from build123d import *

# Parameters (mm, degrees)
BOSS_EXTRUDE1_DEPTH = 40
BOSS_EXTRUDE2_REACH = 105.634
SKETCH2_R           = 18
SKETCH3_R           = 15
SKETCH3_R_2         = 10
BOSS_EXTRUDE3_DEPTH = 18
BOSS_EXTRUDE5_DEPTH = 3
SKETCH5_W           = 20
SKETCH5_H           = 1.869521783
BOSS_EXTRUDE6_DEPTH = 6
SKETCH6_W           = 20
SKETCH6_H           = 1.869521783
BOSS_EXTRUDE7_DEPTH = 6
SKETCH8_W           = 18
SKETCH8_H           = 14
CUT_EXTRUDE1_DEPTH  = 119.321595713
FILLET1_R           = 2
SKETCH9_R           = 4
CUT_EXTRUDE2_DEPTH  = 6


with BuildPart() as part:
    # Sketch1 → Boss-Extrude1 (new body)
    with BuildSketch(Plane(origin=(0, 0, 0), x_dir=(1, 0, 0), z_dir=(0, 1, 0))):
        with BuildLine():
            Line((0, 0), (92, 0))
            Line((92, 0), (92, 6))
            Line((92, 6), (63, 6))
            ThreePointArc((63, 6), (61.585786438, 6.585786438), (61, 8))
            Line((61, 8), (61, 18))
            ThreePointArc((61, 18), (60.414213562, 19.414213562), (59, 20))
            Line((59, 20), (33, 20))
            ThreePointArc((33, 20), (31.585786438, 19.414213562), (31, 18))
            Line((31, 18), (31, 8))
            ThreePointArc((31, 8), (30.414213562, 6.585786438), (29, 6))
            Line((29, 6), (0, 6))
            Line((0, 6), (0, 0))
        make_face()
    extrude(amount=BOSS_EXTRUDE1_DEPTH)

    # Boss-Extrude2: up to this face of the body (flat: up to its plane)
    boss_extrude2_end = Plane(part.part.faces().sort_by_distance((14.5, 20, -6))[0])
    # Sketch2 → Boss-Extrude2 (add, up to the picked face)
    with BuildSketch(Plane(origin=(0, 0, -26), x_dir=(-1, 0, 0), z_dir=(0, 0, -1)), mode=Mode.PRIVATE) as boss_extrude2_sk1:
        with Locations((-46, 20)):
            Circle(SKETCH2_R)
    boss_extrude2_tool1 = split(extrude(boss_extrude2_sk1.sketch, amount=-BOSS_EXTRUDE2_REACH, mode=Mode.PRIVATE), bisect_by=boss_extrude2_end, keep=Keep.BOTH, mode=Mode.PRIVATE)
    add(boss_extrude2_tool1.solids().sort_by(Axis((46, 20, -26), (0, 0, 1)))[0])

    # Sketch3 → Boss-Extrude3 (add)
    with BuildSketch(Plane(origin=(0, 0, -26), x_dir=(-1, 0, 0), z_dir=(0, 0, -1))):
        with Locations((-46, 20)):
            Circle(SKETCH3_R)
        with Locations((-46, 20)):
            Circle(SKETCH3_R_2, mode=Mode.SUBTRACT)
    extrude(amount=BOSS_EXTRUDE3_DEPTH)

    # Sketch4 → Boss-Extrude5 (add, symmetric)
    with BuildSketch(Plane(origin=(0, 20, 0), x_dir=(-1, 0, 0), z_dir=(0, -1, 0))):
        Polygon((-61.98666838, 26), (-83, 6), (-61.98666838, 6), align=None)
        Polygon((-28.035534547, 26), (-9, 6), (-28.035534547, 6), align=None)
    extrude(amount=BOSS_EXTRUDE5_DEPTH, both=True)

    # Sketch5 → Boss-Extrude6 (add)
    with BuildSketch(Plane(origin=(28.035534547, 0, 0), x_dir=(0, 0, -1), z_dir=(1, 0, 0))):
        with Locations((16, 17.934760891)):
            Rectangle(SKETCH5_W, SKETCH5_H)
    extrude(amount=BOSS_EXTRUDE6_DEPTH)

    # Sketch6 → Boss-Extrude7 (add)
    with BuildSketch(Plane(origin=(28.035534547, 0, 0), x_dir=(0, 0, -1), z_dir=(1, 0, 0))):
        with Locations((16, 22.065239109)):
            Rectangle(SKETCH6_W, SKETCH6_H)
    extrude(amount=BOSS_EXTRUDE7_DEPTH)

    # Sketch8 → Cut-Extrude1 (cut, through all)
    with BuildSketch(Plane(origin=(0, 60, 0), x_dir=(1, 0, 0), z_dir=(0, 1, 0))):
        with Locations((46, 7)):
            Rectangle(SKETCH8_W, SKETCH8_H)
    extrude(amount=-CUT_EXTRUDE1_DEPTH, mode=Mode.SUBTRACT)

    # Fillet1
    fillet1_edges = [part.edges().sort_by_distance(p)[0] for p in [
        (92, 40, -3),
        (92, 0, -3),
        (0, 0, -3),
        (0, 40, -3),
    ]]
    fillet(fillet1_edges, radius=FILLET1_R)

    # Sketch9 → Cut-Extrude2 (cut)
    with BuildSketch(Plane.XY):
        with Locations((86, 6)):
            Circle(SKETCH9_R)
        with Locations((85.806998085, 34)):
            Circle(SKETCH9_R)
        with Locations((6, 34)):
            Circle(SKETCH9_R)
        with Locations((6, 6)):
            Circle(SKETCH9_R)
    extrude(amount=-CUT_EXTRUDE2_DEPTH, mode=Mode.SUBTRACT)


solid = part.part
Can you work these out from the model? Positions are in its coordinate system, mm. A direction names the side the tool comes from. Round coordinates to 2 decimals unless told otherwise and drop trailing zeros. Loops run counter-clockwise (first coordinate to the right, second up) from the corner with the lowest first, then second, coordinate; pieces in that order, holes last. Notation, with made-up numbers: (-30, -1) - (-7, -1) arc R13 cw to (-7, 9) - close; hole circle Ø6 at (-40, 73). An arc over 180 degrees is marked (long way). Answer in a Markdown table with one row per item. Add a question column.
Q1. For pin 1 Ø10 at (y, z) = (29.5, -15) entering from +X; pin 2 Ø14.5 at (x, y) = (44.5, 24) entering from +Z; pin 3 Ø14.5 at (x, z) = (73.5, -15) entering from +Y; pin 4 Ø7 at (x, y) = (86, 6) entering from +Z, each with a flat end and sliding along its axis, tell me the tip position at first contact or that it passes through.
Q2. We'd pull the mould along Y, two halves only. Please class faces 1 (the flat face through (69, 23, -11)), 2 (the cylindrical face through (5.479, 37.966, -2.958)), 3 (the flat face through (78, 15, -6)): pulls with the +Y half, pulls with the -Y half, needs draft (parallel to the pull), parting line crosses it, or undercut.
Q3. I want a section at B-B on y = 34. Count the separate pieces of the cut face and the enclosed holes in it, and give its area (3 significant figures).
Q4. I need wall thicknesses on L1, parallel to Y at x = 6, z = -2; L2, parallel to X at y = 13, z = -2.5; L3, parallel to Z at x = 28, y = 38.5. Which ranges of each line are inside material? Lowest first, please.
Q5. Which directions (+Z, -Z, +X, -X, +Y, -Y) give clear straight access to the entire face, cutting with the end or side of a thin tool? Please do faces 4 (the cylindrical face through (30.43, 5.38, -6.6)), 5 (the flat face through (46, 39, -20)), 6 (the cylindrical face through (30.56, 10.75, -20.58)), 7 (the cylindrical face through (60.43, 34.9, -19.4)).
Q6. I want a section at C-C on z = -10. List the corners of the cut face in (x, y) for me.
Q7. I want a section at A-A on x = 6. List the corners of the cut face in (y, z) for me.
Q8. I want a section at D-D on x = 46. List the corners of the cut face in (y, z) for me, and give its area (3 significant figures).
A:
| question | item | result |
|---|---|---|
| 1 | pin 1 | x = 63.43 |
| 1 | pin 2 | z = -14 |
| 1 | pin 3 | y = 23 |
| 1 | pin 4 | through |
| 2 | face 1 | pulls with the +Y half |
| 2 | face 2 | undercut |
| 2 | face 3 | needs draft |
| 3 | separate pieces | 3 |
| 3 | enclosed holes | 0 |
| 3 | area | 954 mm^2 |
| 4 | L1 | 0 to 2, 10 to 30, 38 to 40 |
| 4 | L2 | 0 to 37, 55 to 92 |
| 4 | L3 | -6 to 0 |
| 5 | face 4 | -Z, -X, -Y |
| 5 | face 5 | -Z, +Y |
| 5 | face 6 | -Z |
| 5 | face 7 | -Z, +X, +Y |
| 6 | outline | (12.81, 17) - (28.25, 17) arc R18 ccw to (31, 10.05) - (31, 0) - (37, 0) - (37, 40) - (31, 40) - (31, 29.95) arc R18 ccw to (28.25, 23) - (12.81, 23) - close; (55, 0) - (61, 0) - (61, 10.05) arc R18 ccw to (63.75, 17) - (78.8, 17) - (78.8, 23) - (63.75, 23) arc R18 ccw to (61, 29.95) - (61, 40) - (55, 40) - close |
| 7 | outline | (0, -6) - (2, -6) - (2, 0) - (0, 0) - close; (10, -6) - (30, -6) - (30, 0) - (10, 0) - close; (38, -6) - (40, -6) - (40, 0) - (38, 0) - close |
| 8 | outline | (0, -20) - (2, -20) - (2, -26) - (5, -26) - (5, -44) - (10, -44) - (10, -26) - (30, -26) - (30, -44) - (35, -44) - (35, -26) - (38, -26) - (38, -20) - (40, -20) - (40, -14) - (0, -14) - close |
| 8 | area | 636 mm^2 |
